CAD build for the part. Positions are in the model's coordinates, mm. Round coordinates to 2 decimals unless told otherwise and drop trailing zeros. Loops run counter-clockwise (first coordinate to the right, second up) from the corner with the lowest first, then second, coordinate; pieces in that order, holes last.
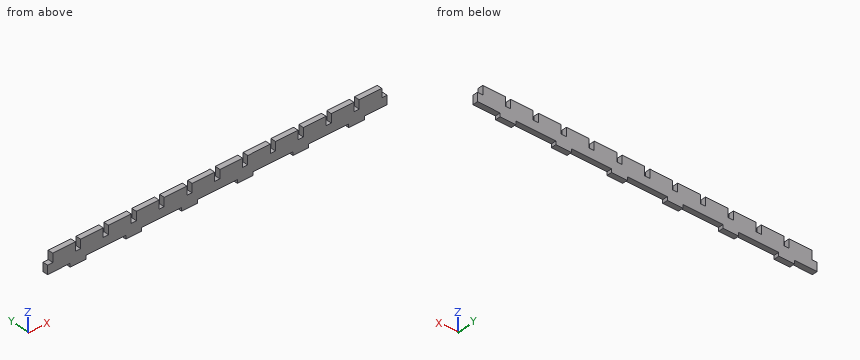
from build123d import *

# Parameters (mm, degrees)
F0_W     = 3
F0_H     = 2
F0_W_2   = 1.5
F0_H_2   = 5
F1_DEPTH = 3


with BuildPart() as f1:
    # F0 (on Front) → F1 (new body)
    with BuildSketch(Plane.XZ):
        Polygon((1.5, 5), (1.5, 0), (11.5, 0), (14.5, 0), (14.5, 5), (14.5, 10), (11.5, 10), (1.5, 10), align=None)
        Polygon((17.5, 5), (17.5, 0), (20.5, 0), (30.5, 0), (30.5, 5), (30.5, 10), (20.5, 10), (17.5, 10), align=None)
        with Locations((45, -1)):
            Rectangle(F0_W, F0_H)
        with Locations((51, -1)):
            Rectangle(F0_W, F0_H)
        with Locations((77, -1)):
            Rectangle(F0_W, F0_H)
        with Locations((83, -1)):
            Rectangle(F0_W, F0_H)
        with Locations((109, -1)):
            Rectangle(F0_W, F0_H)
        with Locations((115, -1)):
            Rectangle(F0_W, F0_H)
        with Locations((141, -1)):
            Rectangle(F0_W, F0_H)
        with Locations((147, -1)):
            Rectangle(F0_W, F0_H)
        with Locations((173, -1)):
            Rectangle(F0_W, F0_H)
        with Locations((179, -1)):
            Rectangle(F0_W, F0_H)
        Polygon((33.5, 5), (33.5, 0), (43.5, 0), (46.5, 0), (46.5, 5), (46.5, 10), (33.5, 10), align=None)
        Polygon((49.5, 5), (49.5, 0), (52.5, 0), (62.5, 0), (62.5, 5), (62.5, 10), (49.5, 10), align=None)
        Polygon((78.5, 10), (65.5, 10), (65.5, 5), (65.5, 0), (75.5, 0), (78.5, 0), (78.5, 5), align=None)
        Polygon((94.5, 10), (81.5, 10), (81.5, 5), (81.5, 0), (84.5, 0), (94.5, 0), (94.5, 5), align=None)
        Polygon((110.5, 10), (97.5, 10), (97.5, 5), (97.5, 0), (107.5, 0), (110.5, 0), (110.5, 5), align=None)
        Polygon((126.5, 10), (113.5, 10), (113.5, 5), (113.5, 0), (116.5, 0), (126.5, 0), (126.5, 5), align=None)
        Polygon((142.5, 10), (129.5, 10), (129.5, 5), (129.5, 0), (139.5, 0), (142.5, 0), (142.5, 5), align=None)
        Polygon((158.5, 10), (145.5, 10), (145.5, 5), (145.5, 0), (148.5, 0), (158.5, 0), (158.5, 5), align=None)
        Polygon((171.5, 10), (161.5, 10), (161.5, 5), (161.5, 0), (171.5, 0), (174.5, 0), (174.5, 5), (174.5, 10), align=None)
        Polygon((180.5, 10), (177.5, 10), (177.5, 5), (177.5, 0), (180.5, 0), (190.5, 0), (190.5, 5), (190.5, 10), align=None)
        with Locations((0.75, 2.5)):
            Rectangle(F0_W_2, F0_H_2)
        with Locations((-0.75, 2.5)):
            Rectangle(F0_W_2, F0_H_2)
        with Locations((16, -1)):
            Rectangle(F0_W, F0_H)
        with Locations((16, 2.5)):
            Rectangle(F0_W, F0_H_2)
        with Locations((32, 2.5)):
            Rectangle(F0_W, F0_H_2)
        with Locations((48, -1)):
            Rectangle(F0_W, F0_H)
        with Locations((48, 2.5)):
            Rectangle(F0_W, F0_H_2)
        with Locations((13, -1)):
            Rectangle(F0_W, F0_H)
        with Locations((19, -1)):
            Rectangle(F0_W, F0_H)
        with Locations((64, 2.5)):
            Rectangle(F0_W, F0_H_2)
        with Locations((80, 2.5)):
            Rectangle(F0_W, F0_H_2)
        with Locations((80, -1)):
            Rectangle(F0_W, F0_H)
        with Locations((96.75, 2.5)):
            Rectangle(F0_W_2, F0_H_2)
        with Locations((112, 2.5)):
            Rectangle(F0_W, F0_H_2)
        with Locations((112, -1)):
            Rectangle(F0_W, F0_H)
        with Locations((128, 2.5)):
            Rectangle(F0_W, F0_H_2)
        with Locations((144, 2.5)):
            Rectangle(F0_W, F0_H_2)
        with Locations((144, -1)):
            Rectangle(F0_W, F0_H)
        with Locations((160, 2.5)):
            Rectangle(F0_W, F0_H_2)
        with Locations((95.25, 2.5)):
            Rectangle(F0_W_2, F0_H_2)
        with Locations((176, 2.5)):
            Rectangle(F0_W, F0_H_2)
        with Locations((176, -1)):
            Rectangle(F0_W, F0_H)
        with Locations((191.25, 2.5)):
            Rectangle(F0_W_2, F0_H_2)
        with Locations((192.75, 2.5)):
            Rectangle(F0_W_2, F0_H_2)
    extrude(amount=F1_DEPTH)


solid = f1.part
Item 1: Flat gauge pins, fed straight in: P1, Ø1.5, axis at x = 128.5, y = -1.5, coming from the +Z side; P2, Ø0.9, axis at x = 65.5, y = -1.5, coming from the -Z side; P3, Ø0.9, axis at y = -2, z = 7.5, coming from the +X side; P4, Ø3, axis at x = 113, z = 6.5, coming from the -Y side. Where does each tip first touch, or does it go through?
Verdict:
P1: stops at z = 5
P2: stops at z = 0
P3: stops at x = 190.5
P4: stops at y = -3
Item 2: Cut at A-A (x = 103). List the corners of the cut face in (y, z), plus the area to 3 significant figures.
Verdict:
outline: (-3, 0) - (0, 0) - (0, 10) - (-3, 10) - close
area: 30.0 mm2
Item 3: Wall check: L1, parallel to X at y = -2.4, z = -0.5; L2, parallel to Z at x = 53.5, y = -2.4. Give the ranges that are in metal, low to high.
Verdict:
L1: x = 11.5 to 20.5, 43.5 to 52.5, 75.5 to 84.5, 107.5 to 116.5, 139.5 to 148.5, 171.5 to 180.5
L2: z = 0 to 10
